Here's how the part is built. I have some questions about the finished solid (model axes, mm). A direction names the side the tool comes from. Round coordinates to 2 decimals unless told otherwise and drop trailing zeros. Loops run counter-clockwise (first coordinate to the right, second up) from the corner with the lowest first, then second, coordinate; pieces in that order, holes last. Notation, with made-up numbers: M 54,6.25 L 84,6.25 A26 ccw 84,22.25 Z; hole C 86,44.25 d7. An arc over 180 degrees is marked long. Answer as a JSON object with one key per item and string values.
from build123d import *

# Parameters (mm, degrees)
SKETCH2_R           = 2.55
SKETCH2_W           = 30
SKETCH2_H           = 15
BOSS_EXTRUDE1_DEPTH = 36
SKETCH3_R           = 4.3
CUT_EXTRUDE1_DEPTH  = 30.6
SKETCH4_R           = 4.05
CUT_EXTRUDE2_DEPTH  = 31.6
FILLET1_R           = 5
CHAMFER1_SIZE       = 1
SKETCH8_R           = 2.55
CUT_EXTRUDE3_DEPTH  = 10
SKETCH9_R           = 3.4
SKETCH9_R_2         = 2.55
BOSS_EXTRUDE3_DEPTH = 1.76
CHAMFER3_SIZE       = 1
CHAMFER4_SIZE       = 1


with BuildPart() as part:
    # Sketch2 → Boss-Extrude1 (new body)
    # profile 1 of 2: a face of its own
    with BuildSketch(Plane.XY):
        Polygon((-326.5, 320), (-311.5, 320), (-311.5, 345), (-311.5, 360), (-326.5, 360), align=None)
        with Locations((-319, 327)):
            Circle(SKETCH2_R, mode=Mode.SUBTRACT)
        with Locations((-319, 352.5)):
            Circle(SKETCH2_R, mode=Mode.SUBTRACT)
    # profile 2 of 2: a face of its own
    with BuildSketch(Plane.XY):
        with Locations((-296.5, 352.5)):
            Rectangle(SKETCH2_W, SKETCH2_H)
        with Locations((-288.5, 352.5)):
            Circle(SKETCH2_R, mode=Mode.SUBTRACT)
    extrude(amount=BOSS_EXTRUDE1_DEPTH)

    # Sketch3 → Cut-Extrude1 (cut)
    with BuildSketch(Plane.XY.offset(36)):
        with Locations((-319, 352.5)):
            Circle(SKETCH3_R)
        with Locations((-319, 327)):
            Circle(SKETCH3_R)
        with Locations((-288.5, 352.5)):
            Circle(SKETCH3_R)
    extrude(amount=-CUT_EXTRUDE1_DEPTH, mode=Mode.SUBTRACT)

    # Sketch4 → Cut-Extrude2 (cut)
    with BuildSketch(Plane(origin=(0, 0, 0), x_dir=(-1, 0, 0), z_dir=(0, 0, -1))):
        with Locations((303.5, 352.5)):
            Circle(SKETCH4_R)
        Polygon((307.55, 354.83826859), (303.5, 357.17653718), (299.45, 354.83826859), (299.45, 350.16173141), (303.5, 347.82346282), (307.55, 350.16173141), align=None)
    extrude(amount=-CUT_EXTRUDE2_DEPTH, mode=Mode.SUBTRACT)

    # Fillet1
    fillet1_edges = [part.edges().sort_by_distance(p)[0] for p in [
        (-311.5, 345, 18),
        (-281.5, 345, 18),
        (-281.5, 360, 18),
        (-311.5, 320, 18),
        (-326.5, 320, 18),
        (-326.5, 360, 18),
    ]]
    fillet(fillet1_edges, radius=FILLET1_R)

    # Chamfer1
    chamfer1_edges = [part.edges().sort_by_distance(p)[0] for p in [
        (-292.8, 352.5, 36),
        (-323.3, 327, 36),
        (-323.3, 352.5, 36),
    ]]
    chamfer(chamfer1_edges, length=CHAMFER1_SIZE)

    # Sketch8 → Cut-Extrude3 (cut)
    with BuildSketch(Plane(origin=(0, 0, 31.6), x_dir=(-1, 0, 0), z_dir=(0, 0, -1))):
        with Locations((303.5, 352.5)):
            Circle(SKETCH8_R)
    extrude(amount=-CUT_EXTRUDE3_DEPTH, mode=Mode.SUBTRACT)

    # Sketch9 → Boss-Extrude3 (add)
    with BuildSketch(Plane.XY.offset(36)):
        with Locations(Location((-303.5, 352.5, 0), (0, 0, 180))):
            Circle(SKETCH9_R)
        with Locations(Location((-303.5, 352.5, 0), (0, 0, 180))):
            Circle(SKETCH9_R_2, mode=Mode.SUBTRACT)
    extrude(amount=BOSS_EXTRUDE3_DEPTH)

    # Chamfer3
    chamfer3_edges = [part.edges().sort_by_distance(p)[0] for p in [
        (-300.1, 352.5, 36),
    ]]
    chamfer(chamfer3_edges, length=CHAMFER3_SIZE)

    # Chamfer4
    chamfer4_edges = [part.edges().sort_by_distance(p)[0] for p in [
        (-305.525, 348.992597115, 0),
        (-307.55, 352.5, 0),
        (-305.525, 356.007402885, 0),
        (-301.475, 356.007402885, 0),
        (-299.45, 352.5, 0),
        (-301.475, 348.992597115, 0),
    ]]
    chamfer(chamfer4_edges, length=CHAMFER4_SIZE)


solid = part.part
Item 1: I'm going to push flat-ended pins straight in: pin 1 Ø8 at (x, z) = (-301.5, 12) entering from -Y; pin 2 Ø7.5 at (y, z) = (335, 26) entering from +X; pin 3 Ø3 at (x, y) = (-302, 354.5) entering from -Z. Where does each tip first touch, or does it pass through?
Resolved:
{"pin 1": "y = 345", "pin 2": "x = -311.5", "pin 3": "z = 31.6"}
Item 2: On a 3-axis mill with a long thin cutter (end or side, diameter ignored), from which of +Z, -Z, +X, -X, +Y, -Y can I reach the whole of each face in a straight line? I mean faces 4 (the face through (-311.5, 332, 18)), 5 (the face through (-316, 353, 5.4)), 6 (the face through (-301.447, 349.009, 16.086)). Say none if no direction works.
Resolved:
{"face 4": "+Z, -Z, +X, -Y", "face 5": "+Z", "face 6": "-Z"}
Item 3: If we mould it in two halves opening along Y, with no side actions, what happens to faces 1 (the face through (-303, 355, 35)), 2 (the face through (-309, 345, 0)), 3 (the face through (-312.93, 321.5, 18.25))? For each: pulls with the +Y half, pulls with the -Y half, needs draft (parallel to the pull), parting line crosses it, or undercut.
Resolved:
{"face 1": "undercut", "face 2": "needs draft", "face 3": "pulls with the -Y half"}
Item 4: Please list where these lines run through material, in increasing order: probe 1 along X at (y, z) = (352.5, 2); probe 2 along Y at (x, z) = (-319, 14.25); probe 3 along X at (y, z) = (352.5, 17.5). Write a range as from..to.
Resolved:
{"probe 1": "-326.5..-321.55, -316.45..-307.55, -299.45..-291.05, -285.95..-281.5", "probe 2": "320..322.7, 331.3..348.2, 356.8..360", "probe 3": "-326.5..-323.3, -314.7..-307.55, -299.45..-292.8, -284.2..-281.5"}
Item 5: I want a section at A-A, the plane x = -319. Please give me the cut outline in (y, z).
Resolved:
{"outline": "M 320,0 L 324.45,0 L 324.45,5.4 L 322.7,5.4 L 322.7,35 L 321.7,36 L 320,36 Z; M 329.55,0 L 349.95,0 L 349.95,5.4 L 348.2,5.4 L 348.2,35 L 347.2,36 L 332.3,36 L 331.3,35 L 331.3,5.4 L 329.55,5.4 Z; M 355.05,0 L 360,0 L 360,36 L 357.8,36 L 356.8,35 L 356.8,5.4 L 355.05,5.4 Z"}
Item 6: I want a section at C-C, the plane x = -288.5. Please give me the cut outline in (y, z), then the cut area to 3 significant figures.
Resolved:
{"outline": "M 345,0 L 349.95,0 L 349.95,5.4 L 348.2,5.4 L 348.2,35 L 347.2,36 L 345,36 Z; M 355.05,0 L 360,0 L 360,36 L 357.8,36 L 356.8,35 L 356.8,5.4 L 355.05,5.4 Z", "area": "248 mm²"}
Item 7: I want a section at D-D, the plane y = 352.5. State how many separate pieces and enclosed holes the cut face has, then the cut area to 3 significant figures.
Resolved:
{"separate pieces": "4", "enclosed holes": "0", "area": "761 mm²"}
Item 8: I want a section at B-B, the plane y = 327. Please give me the cut outline in (x, z).
Resolved:
{"outline": "M -326.5,0 L -321.55,0 L -321.55,5.4 L -323.3,5.4 L -323.3,35 L -324.3,36 L -326.5,36 Z; M -316.45,0 L -311.5,0 L -311.5,36 L -313.7,36 L -314.7,35 L -314.7,5.4 L -316.45,5.4 Z"}
